Build history of the part. All positions in model axes, mm. Face numbers are marked on the shaded views. A direction names the side the tool comes from. Coordinates: 2 decimals unless noted, no trailing zeros. Write each loop counter-clockwise with the first axis right and the second up, starting at its lowest first coordinate (ties: lowest second). Pieces come first, ordered by that corner, then holes. Notation, with made-up numbers: (59.25, 53) -> (70.25, 53) arc R27 ccw to (70.25, 88) -> close; hole circle Ø8 at (64.25, 5.25). An arc over 180 degrees is marked (long way). Write each question's results on one line, items separated by ' | '. Start each with the question number.
Q1. Saw through at A-A on x = -59. Give the cut face in (y, z), and give its area (3 significant figures).
Q2. Drill centre lines: line 1 (Y direction, x = 15.5, z = 24.5); line 2 (X direction, y = 25, z = 35.5); line 3 (X direction, y = 40, z = 35). Where is each one in solid material? Low to high.
Q3. Tool access for the marked faces 5 and 6: list every direction of +Z, -Z, +X, -X, +Y, -Y with a clear straight run to the whole face (end or side of a thin tool).
Q4. Drop flat-ended pins along their axis: pin 1 Ø5 at (y, z) = (34.5, 26.5) entering from +X; pin 2 Ø5 at (y, z) = (-54, 27) entering from -X; pin 3 Ø8 at (y, z) = (40.5, 33) entering from +X. Give the stop position or say it passes through.
Q5. Saw through at C-C on y = -20. Give the cut face in (x, z).
Q6. Saw through at B-B on z = 29. Give the cut face in (x, y).
Q7. Two-plate mould, pull along Y, no slides. Class the marked faces 1, 2, 3 and 4: released by +Y, released by -Y, zero draft, split by the parting line, or undercut.
from build123d import *

# Parameters (mm, degrees)
F0_R     = 83.7442407906
F1_DEPTH = 38.1
F3_DEPTH = 50.8


with BuildPart() as f1:
    # F0 (on Top) → F1 (new body)
    with BuildSketch(Plane.XY):
        Circle(F0_R)
    extrude(amount=F1_DEPTH)

    # F2 (on face) → F3 (cut)
    with BuildSketch(Plane.XY.offset(38.1)):
        with BuildLine():
            Line((12.6646681265, 15.7748187695), (62.9699063944, 15.7748187695))
            ThreePointArc((62.9699063944, 15.7748187695), (44.7615355408, 47.0155182314), (12.6646681265, 63.6683610578))
            Line((12.6646681265, 63.6683610578), (12.6646681265, 15.7748187695))
        make_face()
        with BuildLine():
            ThreePointArc((12.6646681265, -63.6683610578), (46.9802272386, -44.7985743874), (64.1982079564, -9.6251812305))
            Line((64.1982079564, -9.6251812305), (12.6646681265, -9.6251812305))
            Line((12.6646681265, -9.6251812305), (12.6646681265, -63.6683610578))
        make_face()
        with BuildLine():
            Line((-12.7353318735, 15.7748187695), (-12.7353318735, 63.6542641196))
            ThreePointArc((-12.7353318735, 63.6542641196), (-44.7876221412, 46.990668451), (-62.9699063944, 15.7748187695))
            Line((-62.9699063944, 15.7748187695), (-12.7353318735, 15.7748187695))
        make_face()
        with BuildLine():
            ThreePointArc((-64.1982079564, -9.6251812305), (-47.0050830991, -44.7724935801), (-12.7353318735, -63.6542641196))
            Line((-12.7353318735, -63.6542641196), (-12.7353318735, -9.6251812305))
            Line((-12.7353318735, -9.6251812305), (-64.1982079564, -9.6251812305))
        make_face()
    extrude(amount=-F3_DEPTH, mode=Mode.SUBTRACT)


solid = f1.part
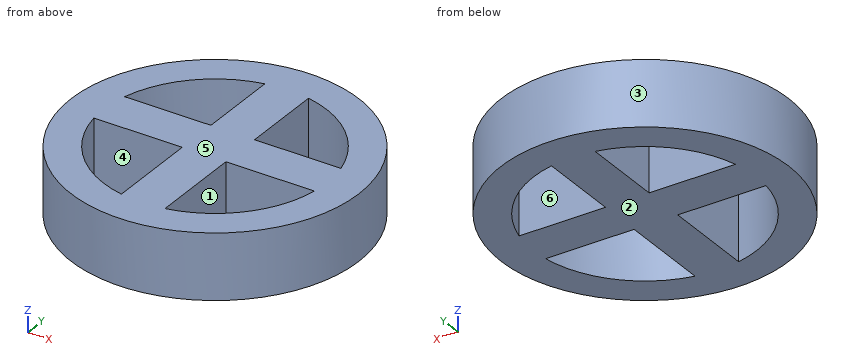
Returned:
1) outline: (-59.43, 0) -> (-27.07, 0) -> (-27.07, 38.1) -> (-59.43, 38.1) -> close; (-9.63, 0) -> (15.77, 0) -> (15.77, 38.1) -> (-9.63, 38.1) -> close; (27.07, 0) -> (59.43, 0) -> (59.43, 38.1) -> (27.07, 38.1) -> close | area: 3,430 mm2
2) line 1: y = -82.3 to -63.04, -9.63 to 15.77, 63.04 to 82.3 | line 2: x = -79.93 to -59.91, -12.74 to 12.66, 59.91 to 79.93 | line 3: x = -73.57 to -51.13, -12.74 to 12.66, 51.13 to 73.57
3) face 5: +Z, +X, -X, +Y, -Y | face 6: +Z, -Z
4) pin 1: stops at x = 77.39 | pin 2: stops at x = -66.04 | pin 3: stops at x = 75.37
5) outline: (-81.32, 0) -> (-61.76, 0) -> (-61.76, 38.1) -> (-81.32, 38.1) -> close; (-12.74, 0) -> (12.66, 0) -> (12.66, 38.1) -> (-12.74, 38.1) -> close; (61.76, 0) -> (81.32, 0) -> (81.32, 38.1) -> (61.76, 38.1) -> close
6) outline: circle Ø167.49 at (0, 0); hole (-64.2, -9.63) arc R64.92 ccw to (-12.74, -63.65) -> (-12.74, -9.63) -> close; hole (-62.97, 15.77) -> (-12.74, 15.77) -> (-12.74, 63.65) arc R64.92 ccw to start; hole (12.66, -63.67) arc R64.92 ccw to (64.2, -9.63) -> (12.66, -9.63) -> close; hole (12.66, 15.77) -> (62.97, 15.77) arc R64.92 ccw to (12.66, 63.67) -> close
7) face 1: undercut | face 2: zero draft | face 3: split by the parting line | face 4: undercut
